Geometry check sheet. Reference: the model listing, model coordinates, mm. A direction names the side the tool comes from. Round coordinates to 2 decimals unless told otherwise and drop trailing zeros. Loops run counter-clockwise (first coordinate to the right, second up) from the corner with the lowest first, then second, coordinate; pieces in that order, holes last. Notation, with made-up numbers: (0, -28.5) -> (51, -28.5) arc R15 cw to (51, -10.5) -> close; hole circle Ø11 at (-36.5, -33.75). An arc over 180 degrees is marked (long way). Use a Markdown table: item, result. Add a question column.
Q1. Set-up check for faces 5 (the face through (52, 33, 28)), 6 (the face through (111, 33, 6)), 7 (the face through (111, 50, 0)): record each of +Z, -Z, +X, -X, +Y, -Y from which the full face is reachable in a straight line by a thin tool's end or side.
Q2. Material ranges on L1, parallel to Y at x = 191.5, z = 5; L2, parallel to Y at x = 30.5, z = 28; L3, parallel to Z at x = 20, y = 32.5, recorded low to high.
Q3. Sectioned sample at B-B, the plane z = 28. Enter the section's corners in (x, y).
Q4. Release check for a two-part mould opening along Y. For faces 1 (the face through (111, 65, 25)), 2 (the face through (111, 35.5, 3)), 3 (the face through (111, 0, 25)), 4 (the face through (225, 33, 25)) record: released by +Y, released by -Y, zero draft, split by the parting line, or undercut.
Q5. Gauge pin test, flat ends, axial feed: P1, Ø9.5, axis at y = 35.5, z = 31, coming from the -X side; P2, Ø6.5, axis at x = 155, y = 31.5, coming from the -Z side. Record the tip position at first contact, or that the pin passes through.
Q6. Sectioned sample at A-A, the plane y = 32.5. Enter the section's corners in (x, z), then the cut area to 3 significant figures.
```python
from build123d import *

# Parameters (mm, degrees)
F1_DEPTH = 225
F2_R     = 9.5
F3_DEPTH = 52


with BuildPart() as f1:
    # F0 (on Right) → F1 (new body)
    with BuildSketch(Plane.YZ):
        Polygon((0, 50), (0, 0), (29.5, 0), (29.5, 6), (32.5, 6), (32.5, 50), align=None)
    extrude(amount=F1_DEPTH)

    # F2 (on face) → F3 (cut)
    with BuildSketch(Plane(origin=(0, 0, 0), x_dir=(0, -1, 0), z_dir=(-1, 0, 0))):
        with Locations((-32.5, 28)):
            Circle(F2_R)
    extrude(amount=-F3_DEPTH, mode=Mode.SUBTRACT)

    # F4: F1 across face


with BuildPart() as f1_1:
    add(f1.part)
    add(f1.part.mirror(Plane(origin=(122.089542, 32.5, 28), x_dir=(-1, 0, 0), z_dir=(0, 1, 0))))


solid = f1_1.part
```
Values:
| question | item | result |
|---|---|---|
| 1 | face 5 | -X |
| 1 | face 6 | -Z, +X, -X |
| 1 | face 7 | -Z, +X, -X, +Y, -Y |
| 2 | L1 | 0 to 29.5, 35.5 to 65 |
| 2 | L2 | 0 to 23, 42 to 65 |
| 2 | L3 | 6 to 18.5, 37.5 to 50 |
| 3 | outline | (0, 0) -> (225, 0) -> (225, 65) -> (0, 65) -> (0, 42) -> (52, 42) -> (52, 23) -> (0, 23) -> close |
| 4 | face 1 | released by +Y |
| 4 | face 2 | undercut |
| 4 | face 3 | released by -Y |
| 4 | face 4 | zero draft |
| 5 | P1 | x = 52 |
| 5 | P2 | z = 0 |
| 6 | outline | (0, 6) -> (225, 6) -> (225, 50) -> (0, 50) -> (0, 37.5) -> (52, 37.5) -> (52, 18.5) -> (0, 18.5) -> close |
| 6 | area | 8,910 mm^2 |
